```python
from build123d import *

# Parameters (mm, degrees)
SKIZZE1_W                        = 65
SKIZZE1_H                        = 50
AUFSATZ_LINEAR_AUSTRAGEN1_DEPTH  = 36
SKIZZE2_W                        = 80
SKIZZE2_H                        = 50
AUFSATZ_LINEAR_AUSTRAGEN2_DEPTH  = 4
SKIZZE3_R                        = 11
SKIZZE3_R_2                      = 1.75
SCHNITT_LINEAR_AUSTRAGEN1_DEPTH  = 4
AUFSATZ_LINEAR_AUSTRAGEN3_DEPTH  = 3.5
AUFSATZ_LINEAR_AUSTRAGEN4_DEPTH  = 3.5
SCHNITT_LINEAR_AUSTRAGEN2_DEPTH  = 27
SKIZZE7_R                        = 11
SCHNITT_LINEAR_AUSTRAGEN3_DEPTH  = 54
SCHNITT_LINEAR_AUSTRAGEN4_DEPTH  = 54
SCHNITT_LINEAR_AUSTRAGEN10_DEPTH = 37
SCHNITT_LINEAR_AUSTRAGEN11_DEPTH = 37


with BuildPart() as part:
    # Skizze1 → Aufsatz-Linear austragen1 (new body)
    with BuildSketch(Plane.XY):
        Rectangle(SKIZZE1_W, SKIZZE1_H)
    extrude(amount=AUFSATZ_LINEAR_AUSTRAGEN1_DEPTH)

    # Skizze2 → Aufsatz-Linear austragen2 (add)
    with BuildSketch(Plane.ZY.offset(32.5)):
        with Locations((40, 0)):
            Rectangle(SKIZZE2_W, SKIZZE2_H)
    extrude(amount=-AUFSATZ_LINEAR_AUSTRAGEN2_DEPTH)

    # Skizze3 → Schnitt-Linear austragen1 (cut)
    with BuildSketch(Plane.ZY.offset(32.5)):
        with Locations(Location((58, 0, 0), (0, 0, 270))):
            Circle(SKIZZE3_R)
        with Locations(Location((73.360257159, 15.75, 0), (0, 0, 270))):
            Circle(SKIZZE3_R_2)
        with Locations(Location((73.360257159, -15.75, 0), (0, 0, 270))):
            Circle(SKIZZE3_R_2)
        with Locations(Location((41.860257159, -15.75, 0), (0, 0, 270))):
            Circle(SKIZZE3_R_2)
        with Locations(Location((41.860257159, 15.75, 0), (0, 0, 270))):
            Circle(SKIZZE3_R_2)
    extrude(amount=-SCHNITT_LINEAR_AUSTRAGEN1_DEPTH, mode=Mode.SUBTRACT)

    # Skizze4 → Aufsatz-Linear austragen3 (add)
    with BuildSketch(Plane(origin=(0, 25, 0), x_dir=(1, 0, 0), z_dir=(0, 1, 0))):
        Polygon((-28.5, -58), (2, -36), (-28.5, -36), align=None)
    extrude(amount=-AUFSATZ_LINEAR_AUSTRAGEN3_DEPTH)

    # Skizze5 → Aufsatz-Linear austragen4 (add)
    with BuildSketch(Plane.XZ.offset(25)):
        Polygon((-28.5, 58), (2, 36), (-28.5, 36), align=None)
    extrude(amount=-AUFSATZ_LINEAR_AUSTRAGEN4_DEPTH)

    # Skizze6 → Schnitt-Linear austragen2 (cut)
    with BuildSketch(Plane.XY.offset(36)):
        with BuildLine():
            Line((-23, 17.5), (5.24803832, 17.5))
            ThreePointArc((5.24803832, 17.5), (6.662251883, 16.914213562), (7.24803832, 15.5))
            Line((7.24803832, 15.5), (7.24803832, -15.5))
            ThreePointArc((7.24803832, -15.5), (6.662251883, -16.914213562), (5.24803832, -17.5))
            Line((5.24803832, -17.5), (-23, -17.5))
            ThreePointArc((-23, -17.5), (-24.414213562, -16.914213562), (-25, -15.5))
            Line((-25, -15.5), (-25, 15.5))
            ThreePointArc((-25, 15.5), (-24.414213562, 16.914213562), (-23, 17.5))
        make_face()
        with BuildLine():
            Line((25, 15.5), (25, -15.5))
            ThreePointArc((25, -15.5), (24.414213562, -16.914213562), (23, -17.5))
            Line((23, -17.5), (11.574569139, -17.5))
            ThreePointArc((11.574569139, -17.5), (10.160355577, -16.914213562), (9.574569139, -15.5))
            Line((9.574569139, -15.5), (9.574569139, 15.5))
            ThreePointArc((9.574569139, 15.5), (10.160355577, 16.914213562), (11.574569139, 17.5))
            Line((11.574569139, 17.5), (23, 17.5))
            ThreePointArc((23, 17.5), (24.414213562, 16.914213562), (25, 15.5))
        make_face()
    extrude(amount=-SCHNITT_LINEAR_AUSTRAGEN2_DEPTH, mode=Mode.SUBTRACT)

    # Skizze7 → Schnitt-Linear austragen3 (cut)
    with BuildSketch(Plane(origin=(32.5, 0, 0), x_dir=(0, 0, -1), z_dir=(1, 0, 0))):
        with Locations((-20, 0)):
            Circle(SKIZZE7_R)
    extrude(amount=-SCHNITT_LINEAR_AUSTRAGEN3_DEPTH, mode=Mode.SUBTRACT)

    # Skizze8 → Schnitt-Linear austragen4 (cut)
    with BuildSketch(Plane(origin=(0, 25, 0), x_dir=(1, 0, 0), z_dir=(0, 1, 0))):
        with BuildLine():
            Line((-14, -9), (-3.639017883, -9))
            ThreePointArc((-3.639017883, -9), (-2.22480432, -9.585786438), (-1.639017883, -11))
            Line((-1.639017883, -11), (-1.639017883, -29))
            ThreePointArc((-1.639017883, -29), (-2.22480432, -30.414213562), (-3.639017883, -31))
            Line((-3.639017883, -31), (-14, -31))
            ThreePointArc((-14, -31), (-25, -20), (-14, -9))
        make_face()
        with BuildLine():
            Line((3.639017883, -9), (14, -9))
            ThreePointArc((14, -9), (25, -20), (14, -31))
            Line((14, -31), (3.639017883, -31))
            ThreePointArc((3.639017883, -31), (2.22480432, -30.414213562), (1.639017883, -29))
            Line((1.639017883, -29), (1.639017883, -11))
            ThreePointArc((1.639017883, -11), (2.22480432, -9.585786438), (3.639017883, -9))
        make_face()
    extrude(amount=-SCHNITT_LINEAR_AUSTRAGEN4_DEPTH, mode=Mode.SUBTRACT)

    # Skizze9 → Schnitt-Linear austragen10 (cut)
    with BuildSketch(Plane.XY.offset(9)):
        with BuildLine():
            Line((-0.5, 14.31913721), (-0.5, -14.31913721))
            ThreePointArc((-0.5, -14.31913721), (-3.5, -17.31913721), (-6.5, -14.31913721))
            Line((-6.5, -14.31913721), (-6.5, 14.31913721))
            ThreePointArc((-6.5, 14.31913721), (-3.5, 17.31913721), (-0.5, 14.31913721))
        make_face()
        with BuildLine():
            Line((24.5, 14.31913721), (24.5, -14.31913721))
            ThreePointArc((24.5, -14.31913721), (21.5, -17.31913721), (18.5, -14.31913721))
            Line((18.5, -14.31913721), (18.5, 14.31913721))
            ThreePointArc((18.5, 14.31913721), (21.5, 17.31913721), (24.5, 14.31913721))
        make_face()
    extrude(amount=-SCHNITT_LINEAR_AUSTRAGEN10_DEPTH, mode=Mode.SUBTRACT)

    # Skizze14 → Schnitt-Linear austragen11 (cut)
    with BuildSketch(Plane.XY.offset(9)):
        with BuildLine():
            Line((1.5, 14.31913721), (1.5, -14.31913721))
            ThreePointArc((1.5, -14.31913721), (-3.5, -19.31913721), (-8.5, -14.31913721))
            Line((-8.5, -14.31913721), (-8.5, 14.31913721))
            ThreePointArc((-8.5, 14.31913721), (-3.5, 19.31913721), (1.5, 14.31913721))
        make_face()
        with BuildLine():
            Line((26.5, 14.31913721), (26.5, -14.31913721))
            ThreePointArc((26.5, -14.31913721), (21.5, -19.31913721), (16.5, -14.31913721))
            Line((16.5, -14.31913721), (16.5, 14.31913721))
            ThreePointArc((16.5, 14.31913721), (21.5, 19.31913721), (26.5, 14.31913721))
        make_face()
    extrude(amount=SCHNITT_LINEAR_AUSTRAGEN11_DEPTH, mode=Mode.SUBTRACT)


solid = part.part
```
The listing builds one solid part. Answer for the finished solid, in the listing's coordinates (mm). A direction names the side the tool comes from. Give positions to 0.01 mm unless a question says otherwise; leave off trailing zeros. Order: outer loops, then holes, each group sorted by start corner. A loop starts at its lowest first (then second) coordinate and runs counter-clockwise, first axis right, second up. Notation, with made-up numbers: (66, 82.5) - (117, 82.5) arc R31 ccw to (117, 120.5) - close; hole circle Ø5 at (15.25, 83). An arc over 180 degrees is marked (long way). Answer in a Markdown table with one row per item. Add a question column.
Q1. The part is cut by section B-B (y = -9.5). Give the number of separate pieces and of enclosed holes in the cut face, then the cut area to 3 significant figures.
Q2. Find the intervals of material crossed by line 1 along Z through (x, y) = (-29.9, 15.75); line 2 along X through (y, z) = (-14, 8); line 3 along Z through (x, y) = (-14.5, -19), in increasing order. Write a range as [from, to].
Q3. The part is cut by section A-A (z = 48.5). Determine the outline of the cut face in (x, y).
Q4. The part is cut by section C-C (x = 20). Determine the outline of the cut face in (y, z).
Q5. Given P1, Ø8, axis at x = 17, y = 7.5, coming from the +Z side; P2, Ø4, axis at y = -12, z = 38.5, coming from the +X side; P3, Ø10, axis at y = -2.5, z = 18, coming from the +X side, each flat-ended and moving along its own axis, determine where each tip first touches the part or whether it passes through.
Q6. The part is cut by section D-D (x = -16.5). Determine the outline of the cut face in (y, z), then the cut area to 3 significant figures.
Q7. For a pull along Z with two mould halves and no side action, classify faces 1 (the cylindrical face through (2.21, -21.2, 9.6)), 2 (the flat face through (9, 0, 36)), 3 (the cylindrical face through (21.57, -17.32, 4.56)) as released by +Z, released by -Z, zero draft, split by the parting line, or undercut.
Q8. Which of the six approach directions +Z, -Z, +X, -X, +Y, -Y give full straight-line access (tool end or side, diameter ignored) to faces 4 (the flat face through (1, 17.5, 29)), 5 (the flat face through (-28.5, 5.9, 67.5)), 6 (the flat face through (-1.639, -22, 20)), 7 (the cylindrical face through (21.43, 17.32, 4.56))?
Determined:
| question | item | result |
|---|---|---|
| 1 | separate pieces | 6 |
| 1 | enclosed holes | 0 |
| 1 | area | 918 mm² |
| 2 | line 1 | z = [0, 40.11], [43.61, 71.61], [75.11, 80] |
| 2 | line 2 | x = [-32.5, -6.5], [-0.5, 18.5], [24.5, 32.5] |
| 2 | line 3 | z = [0, 9.01], [30.99, 36] |
| 3 | outline | (-32.5, -25) - (-15.33, -25) - (-15.33, -21.5) - (-28.5, -21.5) - (-28.5, -5.55) - (-32.5, -5.55) - close; (-32.5, 5.55) - (-28.5, 5.55) - (-28.5, 21.5) - (-15.33, 21.5) - (-15.33, 25) - (-32.5, 25) - close |
| 4 | outline | (-25, 0) - (-16.92, 0) - (-16.92, 9) - (-19.09, 9) - (-19.09, 10.78) - (-25, 10.78) - close; (-25, 29.22) - (-19.09, 29.22) - (-19.09, 36) - (-25, 36) - close; (16.92, 0) - (25, 0) - (25, 10.78) - (19.09, 10.78) - (19.09, 9) - (16.92, 9) - close; (19.09, 29.22) - (25, 29.22) - (25, 36) - (19.09, 36) - close |
| 5 | P1 | stops at z = 9 |
| 5 | P2 | stops at x = -28.5 |
| 5 | P3 | stops at x = -25 |
| 6 | outline | (-25, 0) - (25, 0) - (25, 9.29) - (17.5, 9.29) - (17.5, 9) - (-17.5, 9) - (-17.5, 9.29) - (-25, 9.29) - close; (-25, 30.71) - (-17.5, 30.71) - (-17.5, 36) - (-21.5, 36) - (-21.5, 49.34) - (-25, 49.34) - close; (17.5, 30.71) - (25, 30.71) - (25, 49.34) - (21.5, 49.34) - (21.5, 36) - (17.5, 36) - close |
| 6 | area | 627 mm² |
| 7 | face 1 | undercut |
| 7 | face 2 | released by +Z |
| 7 | face 3 | zero draft |
| 8 | face 4 | +Z |
| 8 | face 5 | +Z, +X |
| 8 | face 6 | +Y, -Y |
| 8 | face 7 | +Z, -Z |
